```python
from build123d import *

# Parameters (mm, degrees)
SKETCH_1_W           = 36
SKETCH_1_H           = 46
EXTRUDE_1_DEPTH      = 3
EXTRUDE_2_DEPTH      = 8.5
EXTRUDE_2_DEPTH_BACK = 13.5
SKETCH_2_W           = 2.54
SKETCH_2_H           = 20.32
SKETCH_2_W_2         = 16.5
SKETCH_2_H_2         = 16.5
SKETCH_3_W           = 16.5
SKETCH_3_H           = 16.5
EXTRUDE_3_DEPTH      = 3.5
SKETCH_4_R           = 8
EXTRUDE_4_DEPTH      = 14.5
SKETCH_5_R           = 1.325
CUT_EXTRUDE_1_DEPTH  = 14.5
SKETCH_7_W           = 16.5
SKETCH_7_H           = 10.5
CUT_EXTRUDE_2_DEPTH  = 31.5


with BuildPart() as part:
    # 草图1 → 凸台-拉伸1 (new body)
    with BuildSketch(Plane(origin=(0, 0, 0), x_dir=(1, 0, 0), z_dir=(0, 1, 0))):
        Rectangle(SKETCH_1_W, SKETCH_1_H)
    extrude(amount=EXTRUDE_1_DEPTH)

    # 草图2 → 凸台-拉伸2 (add, two sides: drawn at the far end of the back side and taken through both)
    with BuildSketch(Plane(origin=(0, 3, 0), x_dir=(1, 0, 0), z_dir=(0, 1, 0)).offset(-EXTRUDE_2_DEPTH_BACK)):
        with Locations((16.73, -12.84)):
            Rectangle(SKETCH_2_W, SKETCH_2_H)
        with Locations((-16.73, -12.84)):
            Rectangle(SKETCH_2_W, SKETCH_2_H)
        with Locations((0, 14.75)):
            Rectangle(SKETCH_2_W_2, SKETCH_2_H_2)
    extrude(amount=EXTRUDE_2_DEPTH + EXTRUDE_2_DEPTH_BACK)

    # 草图3 → 凸台-拉伸3 (add)
    with BuildSketch(Plane(origin=(0, 11.5, 0), x_dir=(1, 0, 0), z_dir=(0, 1, 0))):
        with Locations((0, 14.75)):
            Rectangle(SKETCH_3_W, SKETCH_3_H)
    extrude(amount=EXTRUDE_3_DEPTH)

    # 草图4 → 凸台-拉伸4 (add)
    with BuildSketch(Plane(origin=(0, 15, 0), x_dir=(1, 0, 0), z_dir=(0, 1, 0))):
        with Locations(Location((0, 14.75, 0), (0, 0, 90))):
            Circle(SKETCH_4_R)
    extrude(amount=EXTRUDE_4_DEPTH)

    # 草图5 → 切除-拉伸1 (cut)
    with BuildSketch(Plane(origin=(0, 3, 0), x_dir=(1, 0, 0), z_dir=(0, 1, 0))):
        with Locations(Location((-14.825, 19.875, 0), (0, 0, 270))):
            Circle(SKETCH_5_R)
        with Locations(Location((14.825, 19.875, 0), (0, 0, 270))):
            Circle(SKETCH_5_R)
    extrude(amount=-CUT_EXTRUDE_1_DEPTH, mode=Mode.SUBTRACT)

    # 草图7 → 切除-拉伸2 (cut)
    with BuildSketch(Plane.ZY.offset(8.25)):
        with Locations((-14.75, -5.25)):
            Rectangle(SKETCH_7_W, SKETCH_7_H)
    extrude(amount=-CUT_EXTRUDE_2_DEPTH, mode=Mode.SUBTRACT)


solid = part.part
```
Geometry check sheet. Reference: the model listing, model coordinates, mm. A direction names the side the tool comes from. Give positions to 0.01 mm unless a question says otherwise; leave off trailing zeros. Order: outer loops, then holes, each group sorted by start corner. A loop starts at its lowest first (then second) coordinate and runs counter-clockwise, first axis right, second up. Notation, with made-up numbers: (42, -14.5) - (82, -14.5) arc R20 cw to (82, 22.5) - close; hole circle Ø9 at (66.25, 69.5). An arc over 180 degrees is marked (long way). Write item = value, one per line. Start each with the question number.
1) Scan lines: L1, parallel to X at y = -8, z = 11; L2, parallel to Z at x = -2.5, y = 3.5; L3, parallel to Y at x = 6, z = -5.5. Record each from-to range of solid material in increasing order.
2) Draft check along Z on faces 5 (the flat face through (0, 6, -23)), 6 (the cylindrical face through (13.53, 1.52, -20.16)), 7 (the flat face through (-17, 11.5, 13)). Enter one of: released by +Z, released by -Z, zero draft, split by the parting line, or undercut.
3) Access from +Z, -Z, +X, -X, +Y, -Y to the whole of each face (thin tool, end or side, straight path). Record for faces 1 (the flat face through (-8.25, 9, -15)), 2 (the flat face through (0, 9, -6.5)), 3 (the flat face through (17, -5, 2.68)), 4 (the flat face through (-17, 7, 2.68)).
4) Section check B-B (z = 6.5). Enter the section's corners in (x, y).
5) Gauge pin test, flat ends, axial feed: pin 1 Ø8 at (y, z) = (24.5, -9.5) entering from +X; pin 2 Ø3 at (x, y) = (17, 7.5) entering from -Z; pin 3 Ø8 at (y, z) = (19.5, -10.5) entering from -X. Record the tip position at first contact, or that the pin passes through.
6) Section check D-D (y = 23.5). Enter the section's corners in (x, z).
7) Section check C-C (x = 0). Enter the section's corners in (y, z), then the cut area to 3 significant figures.
8) Section check A-A (y = -1.5). Enter the section's corners in (x, z), then the cut area to 3 significant figures.
Geometry check:
q1.L1 = -18 to -15.46, 15.46 to 18
q1.L2 = -23 to -6.5
q1.L3 = 0 to 3
q2.face_5 = released by -Z
q2.face_6 = undercut
q2.face_7 = zero draft
q3.face_1 = +Z, -Z, -X, +Y
q3.face_2 = +Z, +X, -X, +Y
q3.face_3 = -Z, +X, -X, -Y
q3.face_4 = -Z, +X, -X, +Y
q4.outline = (-18, -10.5) - (-15.46, -10.5) - (-15.46, 0) - (15.46, 0) - (15.46, -10.5) - (18, -10.5) - (18, 11.5) - (15.46, 11.5) - (15.46, 3) - (-15.46, 3) - (-15.46, 11.5) - (-18, 11.5) - close
q5.pin_1 = 7.9
q5.pin_2 = 2.68
q5.pin_3 = -8
q6.outline = circle Ø16 at (0, -14.75)
q7.outline = (0, -23) - (15, -23) - (15, -22.75) - (29.5, -22.75) - (29.5, -6.75) - (15, -6.75) - (15, -6.5) - (3, -6.5) - (3, 23) - (0, 23) - close
q7.area = 568 mm2
q8.outline = (-18, 2.68) - (-15.46, 2.68) - (-15.46, 23) - (-18, 23) - close; (15.46, 2.68) - (18, 2.68) - (18, 23) - (15.46, 23) - close
q8.area = 103 mm2
